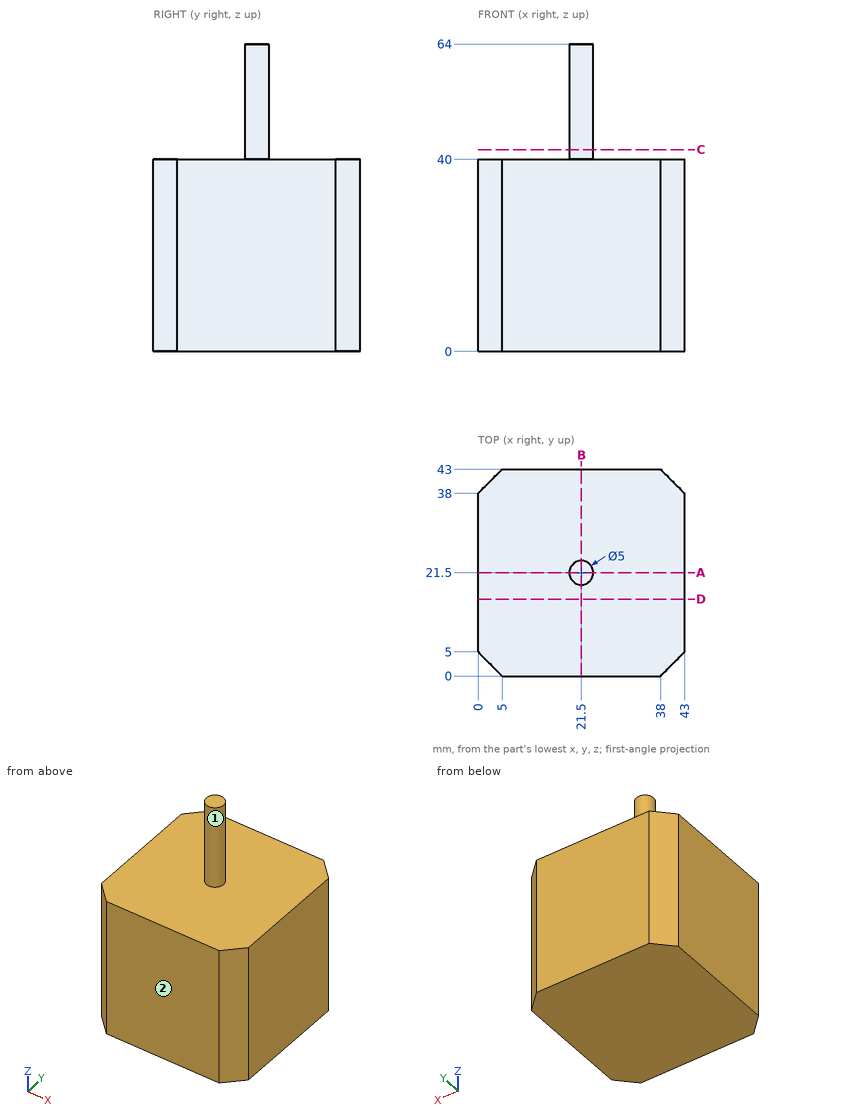
Part print with two shaded views. Sizes in mm from the minimum x, y, z corner. A direction names the side the tool comes from. Round coordinates to 2 decimals unless told otherwise and drop trailing zeros. Order: outer loops, then holes, each group sorted by start corner. A loop starts at its lowest first (then second) coordinate and runs counter-clockwise, first axis right, second up. Notation, with made-up numbers: (53, -35.5) -> (61, -35.5) arc R15 cw to (61, -16.5) -> close; hole circle Ø8 at (-16.5, 0.25). An arc over 180 degrees is marked (long way). Write each question's results on one line, items separated by ' | '.
1. Flat gauge pins, fed straight in: P1, Ø10, axis at x = 5, y = 17, coming from the +Z side; P2, Ø10, axis at x = 36, z = 46, coming from the +Y side; P3, Ø13, axis at x = 14, y = 24, coming from the +Z side; P4, Ø12, axis at x = 21, z = 54, coming from the -Y side. Where does each tip first touch, or does it go through?
Findings below:
P1: stops at z = 40 | P2: passes through | P3: stops at z = 64 | P4: stops at y = 19
2. 3-axis set-ups, long thin cutter, end or side, ignore diameter. For the marked faces 1 and 2: which of +Z, -Z, +X, -X, +Y, -Y reach the whole face in a straight line?
Findings below:
face 1: +Z | face 2: +Z, -Z, +X, -X, -Y
3. Cut at C-C (z = 42). Give the cut face in (x, y), plus the area to 3 significant figures.
Findings below:
outline: circle Ø5 at (21.5, 21.5) | area: 19.6 mm²
4. Cut at D-D (y = 16). Give the cut face in (x, z).
Findings below:
outline: (0, 0) -> (43, 0) -> (43, 40) -> (0, 40) -> close
5. Cut at A-A (y = 21.5). Give the cut face in (x, z), plus the area to 3 significant figures.
Findings below:
outline: (0, 0) -> (43, 0) -> (43, 40) -> (24, 40) -> (24, 64) -> (19, 64) -> (19, 40) -> (0, 40) -> close | area: 1,840 mm²
6. Wall check: line 1 along Z through (x, y) = (37, 33); line 2 along Y through (x, z) = (4.5, 24.5); line 3 along X through (y, z) = (23, 48). Give the ranges that are in metal, low to high. Write a range as [from, to].
Findings below:
line 1: z = [0, 40] | line 2: y = [0.5, 42.5] | line 3: x = [19.5, 23.5]
